Drawing for the job (mm, zero at the part's lowest x, y, z). A direction names the side the tool comes from. Coordinates: 2 decimals unless noted, no trailing zeros. Order: outer loops, then holes, each group sorted by start corner. A loop starts at its lowest first (then second) coordinate and runs counter-clockwise, first axis right, second up.
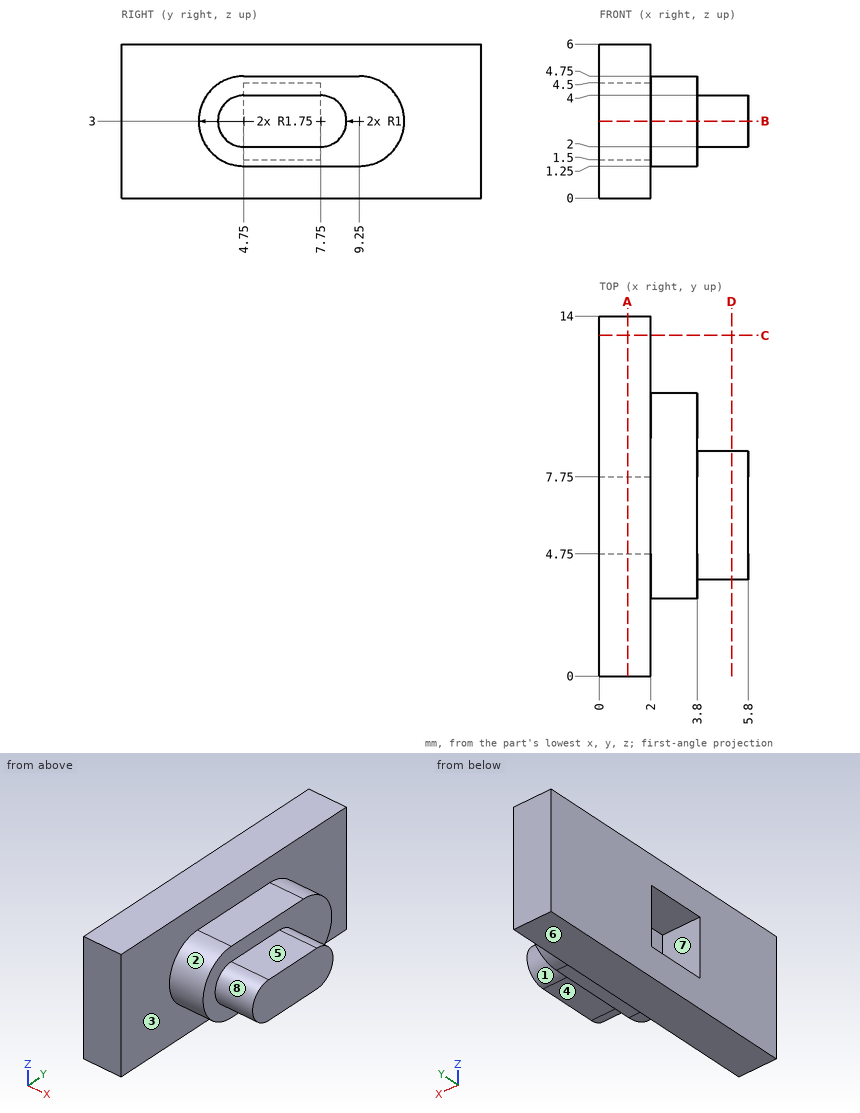
(1) Slice it at C-C, the plane y = 13.25. Give the cut face in (x, z).
(2) Slice it at B-B, the plane z = 3. Give the cut face in (x, y).
(3) Tool access for the marked faces 1, 2, 3, 4 and 5: list every direction of +Z, -Z, +X, -X, +Y, -Y with a clear straight run to the whole face (end or side of a thin tool).
(4) Probe line 1 (X direction, y = 12.25, z = 2.75); line 2 (X direction, y = 10, z = 2); line 3 (Z direction, x = 4.15, y = 7.75). List the from-to ranges inside material, lowest first.
(5) Slice it at A-A, the plane x = 1.1. Give the cut face in (y, z), then the cut area to 3 significant figures.
(6) Pull direction Z, two halves, no side cores. Call the marked faces 6, 7 and 8: +Z half, -Z half, draft (parallel to the pull), parting line (faces both ways), or undercut.
(7) Drop flat-ended pins along their axis: pin 1 (0.6 mm diameter, centred on x = 4.5, y = 6.5, fed in from -Z); pin 2 (0.9 mm diameter, centred on x = 3, y = 6, fed in from +Z); pin 3 (1.6 mm diameter, centred on x = 5, y = 6.5, fed in from +Z). Give the stop position or say it passes through.
(8) Slice it at D-D, the plane x = 5.15. Give the cut face in (y, z), then the cut area to 3 significant figures.
Here are the results:
1. outline: (0, 0) - (2, 0) - (2, 6) - (0, 6) - close
2. outline: (0, 0) - (2, 0) - (2, 3) - (3.8, 3) - (3.8, 3.75) - (5.8, 3.75) - (5.8, 8.75) - (3.8, 8.75) - (3.8, 11) - (2, 11) - (2, 14) - (0, 14) - (0, 7.75) - (2, 7.75) - (2, 4.75) - (0, 4.75) - close
3. face 1: +X, +Y
3. face 2: +X, -Y
3. face 3: +X
3. face 4: -Z, +X, +Y, -Y
3. face 5: +Z, +X, +Y, -Y
4. line 1: x = 0 to 2
4. line 2: x = 0 to 3.8
4. line 3: z = 2 to 4
5. outline: (0, 0) - (14, 0) - (14, 6) - (0, 6) - close; hole (4.75, 1.5) - (7.75, 1.5) - (7.75, 4.5) - (4.75, 4.5) - close
5. area: 75.0 mm2
6. face 6: -Z half
6. face 7: undercut
6. face 8: parting line
7. pin 1: stops at z = 2
7. pin 2: stops at z = 4.75
7. pin 3: stops at z = 4
8. outline: (4.75, 2) - (7.75, 2) arc R1 ccw to (7.75, 4) - (4.75, 4) arc R1 ccw to start
8. area: 9.14 mm2
